from build123d import *

# Parameters (mm, degrees)
SKETCH1_W           = 12.446
SKETCH1_H           = 30.48
SKETCH1_R           = 3
BOSS_EXTRUDE1_DEPTH = 3
SKETCH2_R           = 6.858
BOSS_EXTRUDE2_DEPTH = 16.764


with BuildPart() as part:
    # Sketch1 → Boss-Extrude1 (new body)
    with BuildSketch(Plane(origin=(0, 0, 0), x_dir=(1, 0, 0), z_dir=(0, 1, 0))):
        Rectangle(SKETCH1_W, SKETCH1_H)
        with Locations((0, 8.24)):
            Circle(SKETCH1_R, mode=Mode.SUBTRACT)
    extrude(amount=BOSS_EXTRUDE1_DEPTH)

    # Sketch2 → Boss-Extrude2 (add)
    with BuildSketch(Plane.XY.offset(15.24)):
        with Locations((0, 6.858)):
            Circle(SKETCH2_R)
    extrude(amount=-BOSS_EXTRUDE2_DEPTH)


solid = part.part
Work out the finished part from the listing and answer in its coordinate system (mm). A direction names the side the tool comes from. Give positions to 0.01 mm unless a question says otherwise; leave off trailing zeros. Write each loop counter-clockwise with the first axis right and the second up, starting at its lowest first coordinate (ties: lowest second). Pieces come first, ordered by that corner, then holes. Notation, with made-up numbers: (-13.75, 40) - (17.25, 40) arc R34 cw to (17.25, 70) - close; hole circle Ø10 at (67.5, 81). An arc over 180 degrees is marked (long way). One line per item, written item: value. Start each with the question number.
1. For a pull along X with two mould halves and no side action, classify faces 1 (the flat face through (0, 0, 0)), 2 (the cylindrical face through (-0.391, 1.479, -11.214)), 3 (the flat face through (-6.223, 1, 0)) as +X half, -X half, draft (parallel to the pull), parting line (faces both ways), or undercut.
2. Find section A-A (x = 0). Write down the section's boundary in (y, z), then the cut area to 3 significant figures.
3. Consider probe 1 along X at (y, z) = (1.25, -8.24); probe 2 along Z at (x, y) = (0, 2); probe 3 along Y at (x, z) = (-3.75, -3). Determine where each line is inside the solid, lowest interval first.
4. Find section D-D (y = 11.75). Write down the section's boundary in (x, z), then the cut area to 3 significant figures.
5. Find section B-B (z = -8.24). Write down the section's boundary in (x, y).
6. Given pin 1 (3 mm diameter, centred on x = -4.5, y = 5, fed in from -Z); pin 2 (1.5 mm diameter, centred on y = 2, z = -0.5, fed in from +X); pin 3 (3.5 mm diameter, centred on x = 0, z = -8.24, fed in from -Y); pin 4 (3.5 mm diameter, centred on y = 1, z = -5, fed in from -X), each flat-ended and moving along its own axis, determine where each tip first touches the part or whether it passes through.
7. Find section C-C (x = 4). Write down the section's boundary in (y, z).
8. For faces 4 (the flat face through (0, 7, 15.24)), 5 (the flat face through (0, 8, -1.524)), 6 (the flat face through (6.223, 1, 0)), determine the directions among +Z, -Z, +X, -X, +Y, -Y from which every point of the face is accessible in a straight line to the end or side of a thin tool.
Geometry results:
1. face 1: draft
1. face 2: undercut
1. face 3: -X half
2. outline: (0, -15.24) - (3, -15.24) - (3, -11.24) - (0, -11.24) - close; (0, -5.24) - (3, -5.24) - (3, -1.52) - (13.72, -1.52) - (13.72, 15.24) - (0, 15.24) - close
2. area: 253 mm2
3. probe 1: -6.22 to -3, 3 to 6.22
3. probe 2: -15.24 to -11.24, -5.24 to 15.24
3. probe 3: 0 to 3
4. outline: (-4.81, -1.52) - (4.81, -1.52) - (4.81, 15.24) - (-4.81, 15.24) - close
4. area: 161 mm2
5. outline: (-6.22, 0) - (-3, 0) - (-3, 3) - (-6.22, 3) - close; (3, 0) - (6.22, 0) - (6.22, 3) - (3, 3) - close
6. pin 1: z = -1.52
6. pin 2: x = 6.22
6. pin 3: through
6. pin 4: x = -6.22
7. outline: (0, -15.24) - (3, -15.24) - (3, -1.52) - (12.43, -1.52) - (12.43, 15.24) - (0, 15.24) - close
8. face 4: +Z, +X, -X, +Y, -Y
8. face 5: -Z, +X, -X, +Y
8. face 6: +Z, -Z, +X, -Y
